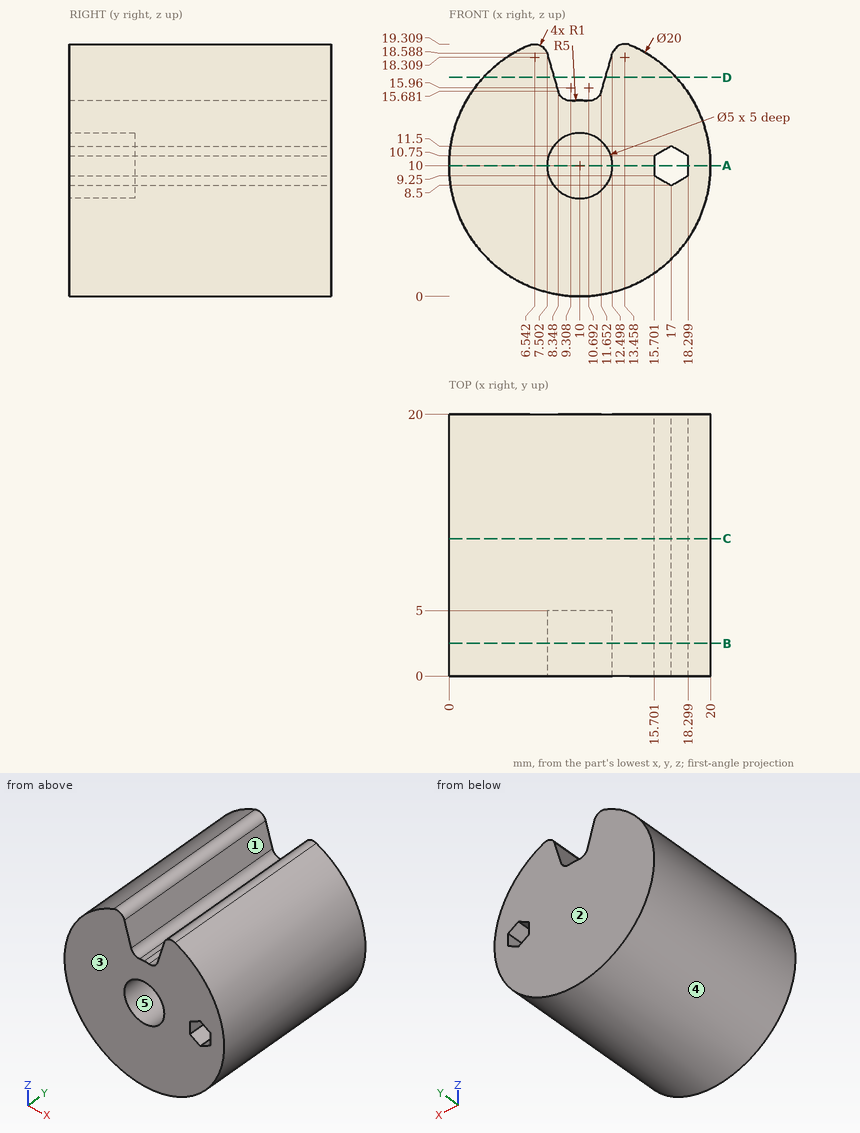
For this review, use the dimensioned drawing (mm, ordinates from the lowest corner) and the shaded views. A direction names the side the tool comes from. Coordinates: 2 decimals unless noted, no trailing zeros. Loops run counter-clockwise (first coordinate to the right, second up) from the corner with the lowest first, then second, coordinate; pieces in that order, holes last. Notation, with made-up numbers: (-34, -6.75) -> (-16, -6.75) arc R25 cw to (-16, 6.25) -> close; hole circle Ø7 at (25, 82). An arc over 180 degrees is marked (long way). Use a Markdown table: item, result. Add a question column.
Item 1: Machinability: for the marked faces 1 and 2, which of the approach directions +Z, -Z, +X, -X, +Y, -Y give a long, thin tool a straight path to every point of the face, cutting with its end or side? Answer none if there is none.
Item 2: We need section B-B, the plane y = 2.5. Write out the cut boundary in (x, z), and give its area (3 significant figures).
Item 3: We need section D-D, the plane z = 16.75. Write out the cut boundary in (x, y), and give its area (3 significant figures).
Item 4: Wall thickness on L1, parallel to X at y = 16.5, z = 16.5; L2, parallel to X at y = 8, z = 15.25 (1 decimal); L3, parallel to Z at x = 5, y = 9.5: over which ranges is each line inside the solid? List them lowest first. Write a range as from..to.
Item 5: We need section A-A, the plane z = 10. Write out the cut boundary in (x, y), and give its area (3 significant figures).
Item 6: Clearance check with flat-ended pins moving along their axes: P1, Ø1.5, axis at x = 2, y = 9, coming from the +Z side; P2, Ø6, axis at y = 11, z = 14, coming from the -X side; P3, Ø1, axis at x = 11, y = 17, coming from the +Z side. State where each tip first meets the part, or that it passes through.
Item 7: The part is to be moulded in two halves that separate along X. For the marked faces 3, 4 and 5, say which applies: +X half, -X half, draft (parallel to the pull), parting line (faces both ways), or undercut.
Item 8: We need section C-C, the plane y = 10.5. Write out the cut boundary in (x, z).
Numbers:
| question | item | result |
|---|---|---|
| 1 | face 1 | +Z, +Y, -Y |
| 1 | face 2 | +Z, -Z, +X, -X, +Y |
| 2 | outline | (6.16, 19.23) arc R10 ccw (long way) to (13.84, 19.23) arc R1 ccw to (12.5, 18.59) -> (11.65, 15.68) arc R1 cw to (10.58, 14.97) arc R5 ccw to (9.42, 14.97) arc R1 cw to (8.35, 15.68) -> (7.5, 18.59) arc R1 ccw to start; hole circle Ø5 at (10, 10); hole (15.7, 9.25) -> (17, 8.5) -> (18.3, 9.25) -> (18.3, 10.75) -> (17, 11.5) -> (15.7, 10.75) -> close |
| 2 | area | 267 mm^2 |
| 3 | outline | (2.62, 0) -> (8.04, 0) -> (8.04, 20) -> (2.62, 20) -> close; (11.96, 0) -> (17.38, 0) -> (17.38, 20) -> (11.96, 20) -> close |
| 3 | area | 217 mm^2 |
| 4 | L1 | x = 2.4..8.11, 11.89..17.6 |
| 4 | L2 | x = 1.5..8.6, 11.4..18.5 |
| 4 | L3 | z = 1.34..18.66 |
| 5 | outline | (0, 0) -> (7.5, 0) -> (7.5, 5) -> (12.5, 5) -> (12.5, 0) -> (15.7, 0) -> (15.7, 20) -> (0, 20) -> close; (18.3, 0) -> (20, 0) -> (20, 20) -> (18.3, 20) -> close |
| 5 | area | 323 mm^2 |
| 6 | P1 | stops at z = 16.89 |
| 6 | P2 | stops at x = 0.05 |
| 6 | P3 | stops at z = 15.37 |
| 7 | face 3 | draft |
| 7 | face 4 | parting line |
| 7 | face 5 | undercut |
| 8 | outline | (6.16, 19.23) arc R10 ccw (long way) to (13.84, 19.23) arc R1 ccw to (12.5, 18.59) -> (11.65, 15.68) arc R1 cw to (10.58, 14.97) arc R5 ccw to (9.42, 14.97) arc R1 cw to (8.35, 15.68) -> (7.5, 18.59) arc R1 ccw to start; hole (15.7, 9.25) -> (17, 8.5) -> (18.3, 9.25) -> (18.3, 10.75) -> (17, 11.5) -> (15.7, 10.75) -> close |
